Design review of the part built by this model. Coordinates are the model's own, in mm. A direction names the side the tool comes from. Coordinates: 2 decimals unless noted, no trailing zeros. Write each loop counter-clockwise with the first axis right and the second up, starting at its lowest first coordinate (ties: lowest second). Pieces come first, ordered by that corner, then holes.
Q1. For faces 1 (the cylindrical face through (23.855, -0.923, -4.156)), 2 (the flat face through (50.477, -3, -1)), 3 (the cylindrical face through (4.05, -1.5, 0.07)), 4 (the cylindrical face through (-6.5, -1.08, -4.88)), list the 3-axis set-ups (+Z, -Z, +X, -X, +Y, -Y) from which the entire face can be reached by the end or side of a thin tool; tool diameter is ignored.
Q2. For L1, parallel to X at y = -2.75, z = 1.5; L2, parallel to X at y = 1.25, z = -4; L3, parallel to Z at x = 11, y = 0, list the stretches that pass through material, from the lowest coordinate up.
Q3. For pin 1 Ø0.9 at (y, z) = (0, 0.5) entering from -X; pin 2 Ø1.5 at (x, y) = (15.5, -3.5) entering from +Z; pin 3 Ø3 at (x, y) = (2.5, -3) entering from -Z, all flat-tipped, find the tip position at first contact; note any pin that passes through.
Q4. Take a section at D-D, the plane x = 44. Write out the cut boundary in (y, z), plus the area to 3 significant figures.
Q5. Take a section at B-B, the plane y = 0. Write out the cut boundary in (x, z).
Q6. Take a section at A-A, the plane x = 0. Write out the cut boundary in (y, z), plus the area to 3 significant figures.
Q7. The part is to be moulded in two halves that separate along Z. For faces 5 (the cylindrical face through (-4.26, -2.1, 1.92)), 6 (the flat face through (-3.523, -1, -3)), 7 (the flat face through (16.977, 0, 0)), say which applies: released by +Z, released by -Z, zero draft, split by the parting line, or undercut.
from build123d import *

# Parameters (mm, degrees)
CHAMFER1_SIZE = 0.5
CHAMFER2_SIZE = 0.5


with BuildPart() as part:
    # Sketch1 → Revolve1 (revolve)
    with BuildSketch(Plane.XY):
        Polygon((-8.523357549, 1.5), (-8.523357549, 5), (-5.023357549, 5), (-5.023357549, 2.846083032), (-3.523357549, 2.846083032), (-3.523357549, 4.257689054), (50.476642451, 4.257689054), (50.476642451, 3), (52.476642451, 3), (52.476642451, 3.956427418), (60.476642451, 3.956427418), (60.476642451, 0), (16.976642451, 0), (16.976642451, 1.5), align=None)
    revolve(axis=Axis((-14.970386809, 0, 0), (1, 0, 0)))

    # Chamfer1
    chamfer1_edges = [part.edges().sort_by_distance(p)[0] for p in [
        (-8.523357549, -5, 0),
    ]]
    chamfer(chamfer1_edges, length=CHAMFER1_SIZE)

    # Chamfer2
    chamfer2_edges = [part.edges().sort_by_distance(p)[0] for p in [
        (60.476642451, -3.956427418, 0),
    ]]
    chamfer(chamfer2_edges, length=CHAMFER2_SIZE)


solid = part.part
Responses:
1. face 1: +X
1. face 2: none
1. face 3: -X
1. face 4: +X, -X
2. L1: x = -8.52 to -5.02, -3.52 to 50.48, 52.48 to 60.48
2. L2: x = -8.52 to -5.02, -3.52 to 50.48
2. L3: z = -4.26 to -1.5, 1.5 to 4.26
3. pin 1: stops at x = 16.98
3. pin 2: stops at z = 3.25
3. pin 3: stops at z = -3.98
4. outline: circle Ø8.52 at (0, 0)
4. area: 57.0 mm2
5. outline: (-8.52, -4.5) - (-8.02, -5) - (-5.02, -5) - (-5.02, -2.85) - (-3.52, -2.85) - (-3.52, -4.26) - (50.48, -4.26) - (50.48, -3) - (52.48, -3) - (52.48, -3.96) - (59.98, -3.96) - (60.48, -3.46) - (60.48, 3.46) - (59.98, 3.96) - (52.48, 3.96) - (52.48, 3) - (50.48, 3) - (50.48, 4.26) - (-3.52, 4.26) - (-3.52, 2.85) - (-5.02, 2.85) - (-5.02, 5) - (-8.02, 5) - (-8.52, 4.5) - (-8.52, 1.5) - (16.98, 1.5) - (16.98, -1.5) - (-8.52, -1.5) - close
6. outline: circle Ø8.52 at (0, 0); hole circle Ø3 at (0, 0)
6. area: 49.9 mm2
7. face 5: split by the parting line
7. face 6: zero draft
7. face 7: undercut
